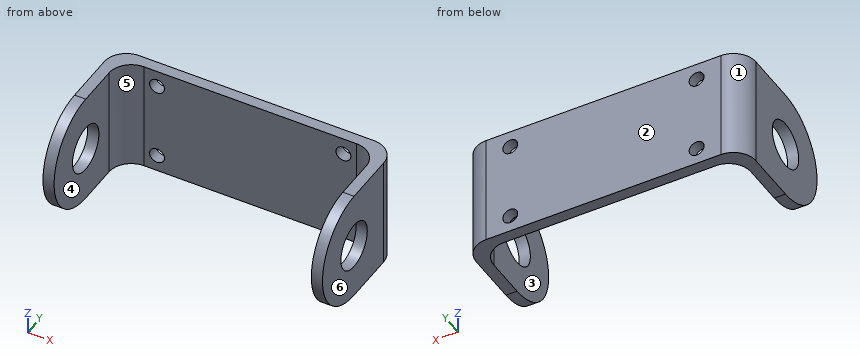
from build123d import *

# Parameters (mm, degrees)
F0_W     = 75
F0_H     = 30
F0_R     = 2
F1_DEPTH = 3
F2_W     = 3
F2_H     = 30
F3_DEPTH = 37
F4_R     = 6.25
F5_DEPTH = 2500
F6_R     = 6


with BuildPart() as f1:
    # F0 (on Front) → F1 (new body)
    with BuildSketch(Plane.XZ):
        Rectangle(F0_W, F0_H)
        with Locations((-25, -10.5)):
            Circle(F0_R, mode=Mode.SUBTRACT)
        with Locations((25, -10.5)):
            Circle(F0_R, mode=Mode.SUBTRACT)
        with Locations((-25, 10.5)):
            Circle(F0_R, mode=Mode.SUBTRACT)
        with Locations((25, 10.5)):
            Circle(F0_R, mode=Mode.SUBTRACT)
    extrude(amount=F1_DEPTH)

    # F2 (on face) → F3 (join)
    with BuildSketch(Plane.XZ.offset(3)):
        with Locations((-36, 0)):
            Rectangle(F2_W, F2_H)
        with Locations((36, 0)):
            Rectangle(F2_W, F2_H)
    extrude(amount=F3_DEPTH)

    # F4 (on face) → F5 (cut)
    with BuildSketch(Plane.YZ.offset(37.5)):
        with Locations((-20, 0)):
            Circle(F4_R)
        with BuildLine():
            ThreePointArc((-20, -15), (-34.945094, 0), (-20, 15))
            Line((-20, 15), (-40, 15))
            Line((-40, 15), (-40, -15))
            Line((-40, -15), (-20, -15))
        make_face()
    extrude(amount=-F5_DEPTH, mode=Mode.SUBTRACT)

    # F6
    f6_edges = [f1.edges().sort_by_distance(p)[0] for p in [
        (37.5, 0, 0),
        (-37.5, 0, 0),
        (-34.5, -3, 0),
        (34.5, -3, 0),
    ]]
    fillet(f6_edges, radius=F6_R)


solid = f1.part
For this review, take the finished solid that the model builds, in its own axes (mm). Face numbers are marked on the shaded views. A direction names the side the tool comes from. Give positions to 0.01 mm unless a question says otherwise; leave off trailing zeros. Loops run counter-clockwise (first coordinate to the right, second up) from the corner with the lowest first, then second, coordinate; pieces in that order, holes last. Notation, with made-up numbers: M 17,29 L 30,29 A15 ccw 30,34 Z; hole C 16,-11.75 d2. An arc over 180 degrees is marked long. Put each result on its own line as item: value. Start each with the question number.
(1) Add section D-D, the plane x = 15.5. Write out the cut boundary in (y, z).
(2) Add section C-C, the plane y = -27. Write out the cut boundary in (x, z), then the cut area to 3 significant figures.
(3) Add section B-B, the plane z = -10.5. Write out the cut boundary in (x, y).
(4) Wall thickness on L1, parallel to Z at x = -25, y = -1; L2, parallel to X at y = -24.5, z = 5.5; L3, parallel to Z at x = 35, y = -20: over which ranges is each line inside the solid? List them lowest first.
(5) Add section A-A, the plane x = 25. Write out the cut boundary in (y, z), then the cut area to 3 significant figures.
(6) Machinability: for the marked faces 5 and 6, which of the approach directions +Z, -Z, +X, -X, +Y, -Y give a long, thin tool a straight path to every point of the face, cutting with its end or side? Answer none if there is none.
(7) The part is to be moulded in two halves that separate along X. For the marked faces 1, 2, 3 and 4, say which applies: +X half, -X half, draft (parallel to the pull), parting line (faces both ways), or undercut.
(8) For pin 1 (8 mm diameter, centred on x = 27.5, z = 5.5, fed in from -Y); pin 2 (2.5 mm diameter, centred on x = -25, z = -10.5, fed in from -Y) (3 decimals); pin 3 (6 mm diameter, centred on x = 21, z = 10.5, fed in from -Y); pin 4 (1.5 mm diameter, centred on y = -4.5, z = -2, fed in from -X), all flat-tipped, find the tip position at first contact; note any pin that passes through.
Result:
1. outline: M -3,-15 L 0,-15 L 0,15 L -3,15 Z
2. outline: M -37.5,-13.24 L -34.5,-13.24 L -34.5,13.24 L -37.5,13.24 Z; M 34.5,-13.24 L 37.5,-13.24 L 37.5,13.24 L 34.5,13.24 Z
2. area: 159 mm^2
3. outline: M -37.5,-30.66 L -34.5,-30.66 L -34.5,-9 A6 cw -28.5,-3 L -27,-3 L -27,0 L -31.5,0 A6 ccw -37.5,-6 Z; M -23,-3 L 23,-3 L 23,0 L -23,0 Z; M 27,-3 L 28.5,-3 A6 cw 34.5,-9 L 34.5,-30.66 L 37.5,-30.66 L 37.5,-6 A6 ccw 31.5,0 L 27,0 Z
4. L1: z = -15 to -12.5, -8.5 to 8.5, 12.5 to 15
4. L2: x = -37.5 to -34.5, 34.5 to 37.5
4. L3: z = -15 to -6.25, 6.25 to 15
5. outline: M -3,-15 L 0,-15 L 0,-12.5 L -3,-12.5 Z; M -3,-8.5 L 0,-8.5 L 0,8.5 L -3,8.5 Z; M -3,12.5 L 0,12.5 L 0,15 L -3,15 Z
5. area: 66.0 mm^2
6. face 5: +Z, -Z, -Y
6. face 6: +Z, -Z, +X, +Y, -Y
7. face 1: -X half
7. face 2: draft
7. face 3: undercut
7. face 4: undercut
8. pin 1: stops at y = -3.8
8. pin 2: passes through
8. pin 3: stops at y = -3
8. pin 4: stops at x = -37.45
